from build123d import *

# Parameters (mm, degrees)
SKETCH1_W           = 48
SKETCH1_H           = 10
BOSS_EXTRUDE1_DEPTH = 1
SKETCH2_W           = 6
SKETCH2_H           = 6
BOSS_EXTRUDE2_DEPTH = 3
SKETCH2_2_W         = 6
SKETCH2_2_H         = 6
BOSS_EXTRUDE3_DEPTH = 3.1
SKETCH4_R           = 1.75
BOSS_EXTRUDE4_DEPTH = 2.9


with BuildPart() as part:
    # Sketch1 → Boss-Extrude1 (new body)
    with BuildSketch(Plane(origin=(0, 0, 0), x_dir=(1, 0, 0), z_dir=(0, 1, 0))):
        Rectangle(SKETCH1_W, SKETCH1_H)
    extrude(amount=BOSS_EXTRUDE1_DEPTH)

    # Sketch2 → Boss-Extrude2 (add)
    with BuildSketch(Plane(origin=(0, 1, 0), x_dir=(1, 0, 0), z_dir=(0, 1, 0))):
        with Locations((-6, 0)):
            Rectangle(SKETCH2_W, SKETCH2_H)
        with Locations((-18, 0)):
            Rectangle(SKETCH2_W, SKETCH2_H)
        with Locations((6, 0)):
            Rectangle(SKETCH2_W, SKETCH2_H)
        with Locations((18, 0)):
            Rectangle(SKETCH2_W, SKETCH2_H)
    extrude(amount=BOSS_EXTRUDE2_DEPTH)

    # Sketch2_2 → Boss-Extrude3 (add)
    with BuildSketch(Plane(origin=(0, 1, 0), x_dir=(1, 0, 0), z_dir=(0, 1, 0))):
        with Locations((-6, 0)):
            Rectangle(SKETCH2_2_W, SKETCH2_2_H)
        with Locations((-18, 0)):
            Rectangle(SKETCH2_2_W, SKETCH2_2_H)
        with Locations((6, 0)):
            Rectangle(SKETCH2_2_W, SKETCH2_2_H)
        with Locations((18, 0)):
            Rectangle(SKETCH2_2_W, SKETCH2_2_H)
    extrude(amount=BOSS_EXTRUDE3_DEPTH)

    # Sketch4 → Boss-Extrude4 (add)
    with BuildSketch(Plane(origin=(0, 4.1, 0), x_dir=(1, 0, 0), z_dir=(0, 1, 0))):
        with Locations(Location((-18, 0, 0), (0, 0, 270))):
            Circle(SKETCH4_R)
        with Locations(Location((18, 0, 0), (0, 0, 270))):
            Circle(SKETCH4_R)
        with Locations(Location((6, 0, 0), (0, 0, 270))):
            Circle(SKETCH4_R)
        with Locations(Location((-6, 0, 0), (0, 0, 270))):
            Circle(SKETCH4_R)
    extrude(amount=BOSS_EXTRUDE4_DEPTH)


solid = part.part
Verification items for the finished model (mm, model axes). A direction names the side the tool comes from. Coordinates: 2 decimals unless noted, no trailing zeros. Order: outer loops, then holes, each group sorted by start corner. A loop starts at its lowest first (then second) coordinate and runs counter-clockwise, first axis right, second up.
1. Sectioned sample at A-A, the plane y = 2. Record the cut outline in (x, z), and give its area (3 significant figures).
Results found:
outline: (-21, -3) - (-15, -3) - (-15, 3) - (-21, 3) - close; (-9, -3) - (-3, -3) - (-3, 3) - (-9, 3) - close; (3, -3) - (9, -3) - (9, 3) - (3, 3) - close; (15, -3) - (21, -3) - (21, 3) - (15, 3) - close
area: 144 mm2
2. Sectioned sample at B-B, the plane x = 18. Record the cut outline in (y, z).
Results found:
outline: (0, -5) - (1, -5) - (1, -3) - (4.1, -3) - (4.1, -1.75) - (7, -1.75) - (7, 1.75) - (4.1, 1.75) - (4.1, 3) - (1, 3) - (1, 5) - (0, 5) - close
3. Set-up check for faces 1 (the face through (15, 3, 0)), 2 (the face through (6, 3, 3)), 3 (the face through (-6, 3, -3)), 4 (the face through (-18, 7, 0)), 5 (the face through (-16.265, 5.53, -0.228)): record each of +Z, -Z, +X, -X, +Y, -Y from which the full face is reachable in a straight line by a thin tool's end or side.
Results found:
face 1: +Z, -Z, +Y
face 2: +Z, +X, -X, +Y
face 3: -Z, +X, -X, +Y
face 4: +Z, -Z, +X, -X, +Y
face 5: +Y
4. Release check for a two-part mould opening along X. For faces 6 (the face through (6, 3, -3)), 7 (the face through (9, 3, 0)), 8 (the face through (-24, 0.5, 0.1)) record: +X half, -X half, draft (parallel to the pull), parting line (faces both ways), or undercut.
Results found:
face 6: draft
face 7: undercut
face 8: -X half
5. Scan lines: line 1 (X direction, y = 4, z = 0); line 2 (X direction, y = 4.5, z = -0.25); line 3 (Z direction, x = 8, y = 3.5). Record each from-to range of solid material in increasing order.
Results found:
line 1: x = -21 to -15, -9 to -3, 3 to 9, 15 to 21
line 2: x = -19.73 to -16.27, -7.73 to -4.27, 4.27 to 7.73, 16.27 to 19.73
line 3: z = -3 to 3
6. Sectioned sample at D-D, the plane y = 4.5. Record the cut outline in (x, z), and give its area (3 significant figures).
Results found:
outline: circle Ø3.5 at (-18, 0); circle Ø3.5 at (-6, 0); circle Ø3.5 at (6, 0); circle Ø3.5 at (18, 0)
area: 38.5 mm2
7. Sectioned sample at C-C, the plane z = 2.25. Record the cut outline in (x, y).
Results found:
outline: (-24, 0) - (24, 0) - (24, 1) - (21, 1) - (21, 4.1) - (15, 4.1) - (15, 1) - (9, 1) - (9, 4.1) - (3, 4.1) - (3, 1) - (-3, 1) - (-3, 4.1) - (-9, 4.1) - (-9, 1) - (-15, 1) - (-15, 4.1) - (-21, 4.1) - (-21, 1) - (-24, 1) - close
8. Go/stop test with flat-tipped pins: pin 1 Ø3.5 at (x, y) = (6.5, 3.5) entering from -Z; pin 2 Ø3.5 at (x, y) = (18, 2.5) entering from -Z; pin 3 Ø1.5 at (y, z) = (3.5, 1.5) entering from +X; pin 4 Ø1.5 at (x, y) = (-6, 3.5) entering from +Z. Record where each tip stops, or that it passes through.
Results found:
pin 1: stops at z = -3
pin 2: stops at z = -5
pin 3: stops at x = 21
pin 4: stops at z = 3
